Can you work these out from the model? Positions are in its coordinate system, mm. Round coordinates to 2 decimals unless told otherwise and drop trailing zeros. One line per item, written item: value. Start each with the question number.
(1) I want a section at A-A on z = 0. Give the number of separate pieces and of enclosed holes in the cut face, plus the area to 3 significant figures.
(2) I'm going to push a flat-ended pin straight in: pin 1 Ø7.5 at (x, z) = (326.175, 0) entering from +Y. Where does the tip first touch, or does it pass through?
(3) If I drill on L1, parallel to Z at x = 323.5, y = -0.25; L2, parallel to Z at x = 175, y = 0, over which ranges is the centre line in solid material (lowest first)? Write a range as from..to.
from build123d import *

# Parameters (mm, degrees)
SKETCH1_W           = 997.65
SKETCH1_H           = 18.3
SKETCH1_R           = 3.25
BOSS_EXTRUDE1_DEPTH = 1


with BuildPart() as part:
    # Sketch1 → Boss-Extrude1 (new, symmetric)
    with BuildSketch(Plane(origin=(0, 0, 0), x_dir=(1, 0, 0), z_dir=(0, 1, 0))):
        Rectangle(SKETCH1_W, SKETCH1_H)
        with Locations(Location((-483.825, 0, 0), (0, 0, 270))):
            Circle(SKETCH1_R, mode=Mode.SUBTRACT)
        with Locations(Location((-453.825, 0, 0), (0, 0, 270))):
            Circle(SKETCH1_R, mode=Mode.SUBTRACT)
        with Locations(Location((-423.825, 0, 0), (0, 0, 270))):
            Circle(SKETCH1_R, mode=Mode.SUBTRACT)
        with Locations(Location((-393.825, 0, 0), (0, 0, 270))):
            Circle(SKETCH1_R, mode=Mode.SUBTRACT)
        with Locations(Location((-363.825, 0, 0), (0, 0, 270))):
            Circle(SKETCH1_R, mode=Mode.SUBTRACT)
        with Locations(Location((-333.825, 0, 0), (0, 0, 270))):
            Circle(SKETCH1_R, mode=Mode.SUBTRACT)
        with Locations(Location((-303.825, 0, 0), (0, 0, 270))):
            Circle(SKETCH1_R, mode=Mode.SUBTRACT)
        with Locations(Location((-273.825, 0, 0), (0, 0, 270))):
            Circle(SKETCH1_R, mode=Mode.SUBTRACT)
        with Locations(Location((-243.825, 0, 0), (0, 0, 270))):
            Circle(SKETCH1_R, mode=Mode.SUBTRACT)
        with Locations(Location((-213.825, 0, 0), (0, 0, 270))):
            Circle(SKETCH1_R, mode=Mode.SUBTRACT)
        with Locations(Location((-183.825, 0, 0), (0, 0, 270))):
            Circle(SKETCH1_R, mode=Mode.SUBTRACT)
        with Locations(Location((-153.825, 0, 0), (0, 0, 270))):
            Circle(SKETCH1_R, mode=Mode.SUBTRACT)
        with Locations(Location((-123.825, 0, 0), (0, 0, 270))):
            Circle(SKETCH1_R, mode=Mode.SUBTRACT)
        with Locations(Location((-93.825, 0, 0), (0, 0, 270))):
            Circle(SKETCH1_R, mode=Mode.SUBTRACT)
        with Locations(Location((-63.825, 0, 0), (0, 0, 270))):
            Circle(SKETCH1_R, mode=Mode.SUBTRACT)
        with Locations(Location((-33.825, 0, 0), (0, 0, 270))):
            Circle(SKETCH1_R, mode=Mode.SUBTRACT)
        with Locations(Location((-3.825, 0, 0), (0, 0, 270))):
            Circle(SKETCH1_R, mode=Mode.SUBTRACT)
        with Locations(Location((26.175, 0, 0), (0, 0, 270))):
            Circle(SKETCH1_R, mode=Mode.SUBTRACT)
        with Locations(Location((56.175, 0, 0), (0, 0, 270))):
            Circle(SKETCH1_R, mode=Mode.SUBTRACT)
        with Locations(Location((86.175, 0, 0), (0, 0, 270))):
            Circle(SKETCH1_R, mode=Mode.SUBTRACT)
        with Locations(Location((116.175, 0, 0), (0, 0, 270))):
            Circle(SKETCH1_R, mode=Mode.SUBTRACT)
        with Locations(Location((146.175, 0, 0), (0, 0, 270))):
            Circle(SKETCH1_R, mode=Mode.SUBTRACT)
        with Locations(Location((176.175, 0, 0), (0, 0, 270))):
            Circle(SKETCH1_R, mode=Mode.SUBTRACT)
        with Locations(Location((206.175, 0, 0), (0, 0, 270))):
            Circle(SKETCH1_R, mode=Mode.SUBTRACT)
        with Locations(Location((236.175, 0, 0), (0, 0, 270))):
            Circle(SKETCH1_R, mode=Mode.SUBTRACT)
        with Locations(Location((266.175, 0, 0), (0, 0, 270))):
            Circle(SKETCH1_R, mode=Mode.SUBTRACT)
        with Locations(Location((296.175, 0, 0), (0, 0, 270))):
            Circle(SKETCH1_R, mode=Mode.SUBTRACT)
        with Locations(Location((326.175, 0, 0), (0, 0, 270))):
            Circle(SKETCH1_R, mode=Mode.SUBTRACT)
        with Locations(Location((356.175, 0, 0), (0, 0, 270))):
            Circle(SKETCH1_R, mode=Mode.SUBTRACT)
        with Locations(Location((386.175, 0, 0), (0, 0, 270))):
            Circle(SKETCH1_R, mode=Mode.SUBTRACT)
        with Locations(Location((416.175, 0, 0), (0, 0, 270))):
            Circle(SKETCH1_R, mode=Mode.SUBTRACT)
        with Locations(Location((446.175, 0, 0), (0, 0, 270))):
            Circle(SKETCH1_R, mode=Mode.SUBTRACT)
        with Locations(Location((476.175, 0, 0), (0, 0, 270))):
            Circle(SKETCH1_R, mode=Mode.SUBTRACT)
    extrude(amount=BOSS_EXTRUDE1_DEPTH, both=True)


solid = part.part
Established:
1. separate pieces: 34
1. enclosed holes: 0
1. area: 1,570 mm2
2. pin 1: y = 1
3. L1: -9.15..-1.85, 1.85..9.15
3. L2: -9.15..-3.03, 3.03..9.15
